Model file for the job. Use its own axes, mm. Coordinates: 2 decimals unless noted, no trailing zeros. Write each loop counter-clockwise with the first axis right and the second up, starting at its lowest first coordinate (ties: lowest second). Pieces come first, ordered by that corner, then holes. Notation, with made-up numbers: M -20.5,25 L 17.5,25 A26 cw 17.5,51 Z; hole C -10.5,89 d2. An arc over 180 degrees is marked long. Use CSV: the item, a comma, the result in double quotes. Start each with the question number.
from build123d import *

# Parameters (mm, degrees)
F0_W          = 40
F0_H          = 40
F1_DEPTH      = 20
F1_DEPTH_BACK = 20
F2_SIZE       = 39.99999


# Not quite as in the source:
# - a fillet or chamfer is up to 0.001 mm smaller than in the source, because OpenCascade refuses the exact size


with BuildPart() as f1:
    # F0 (on Top) → F1 (new body, two sides)
    with BuildSketch(Plane.XY) as f1_sk:
        Rectangle(F0_W, F0_H)
    extrude(amount=F1_DEPTH)
    extrude(f1_sk.sketch, amount=-F1_DEPTH_BACK)

    # F2 (size 40 in the source; OpenCascade refuses exactly that, so slightly less here)
    f2_edges = [f1.edges().sort_by_distance(p)[0] for p in [
        (20, 0, 20),
    ]]
    chamfer(f2_edges, length=F2_SIZE)


solid = f1.part
1) Drop flat-ended pins along their axis: P1, Ø1.5, axis at x = 5, y = -3, coming from the +Z side; P2, Ø2, axis at y = -15.5, z = -5, coming from the +X side; P3, Ø2, axis at y = -10.5, z = 12, coming from the +X side. Give the stop position or say it passes through.
2) Band-saw the part on C-C on x = 17. List the corners of the cut face in (y, z).
3) Wall check: L1, parallel to Z at x = 12.5, y = 15; L2, parallel to X at y = 8.5, z = -3.5; L3, parallel to Z at x = 17.5, y = 12.5. Give the ranges that are in metal, low to high. Write a range as [from, to].
4) Band-saw the part on B-B on z = -15.5. List the corners of the cut face in (x, y), then the cut area to 3 significant figures.
Findings below:
1,P1,"stops at z = -4.25"
1,P2,"stops at x = 6"
1,P3,"stops at x = -11"
2,outline,"M -20,-20 L 20,-20 L 20,-17 L -20,-17 Z"
3,L1,"z = [-20, -12.5]"
3,L2,"x = [-20, 3.5]"
3,L3,"z = [-20, -17.5]"
4,outline,"M -20,-20 L 15.5,-20 L 15.5,20 L -20,20 Z"
4,area,"1,420 mm2"
